Can you work these out from the model? Positions are in its coordinate system, mm. Face numbers are marked on the shaded views. A direction names the side the tool comes from. Round coordinates to 2 decimals unless told otherwise and drop trailing zeros. Order: outer loops, then holes, each group sorted by start corner. A loop starts at its lowest first (then second) coordinate and runs counter-clockwise, first axis right, second up. Notation, with made-up numbers: (2, -37) -> (60, -37) arc R16 ccw to (60, -26) -> close; hole circle Ø5 at (24, 66). An arc over 180 degrees is marked (long way). One line per item, written item: value.
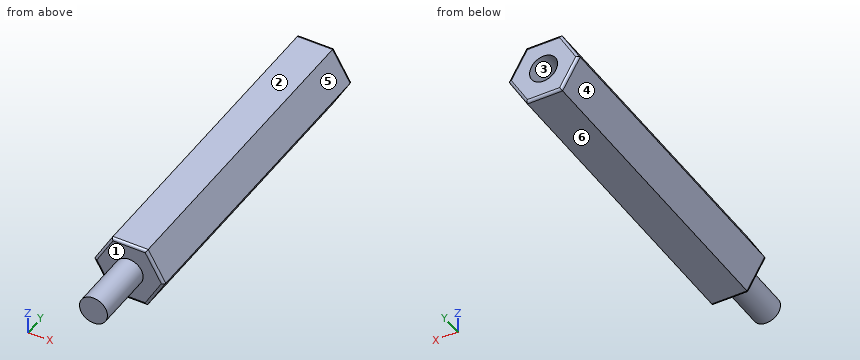
```python
from build123d import *

# Parameters (mm, degrees)
RESSALTO_EXTRUS_O1_DEPTH = 25
FILETE1_R                = 0.2
ESBO_O2_R                = 1.0922
RESSALTO_EXTRUS_O2_DEPTH = 4.76
ESBO_O3_R                = 1.0922
CORTE_EXTRUS_O1_DEPTH    = 4.76


with BuildPart() as part:
    # Esboço1 → Ressalto-extrusão1 (new body)
    with BuildSketch(Plane(origin=(0, 0, 0), x_dir=(1, 0, 0), z_dir=(0, 1, 0))):
        Polygon((2.748187281, 0), (1.374093641, 2.38), (-1.374093641, 2.38), (-2.748187281, 0), (-1.374093641, -2.38), (1.374093641, -2.38), align=None)
    extrude(amount=RESSALTO_EXTRUS_O1_DEPTH)

    # Filete1
    filete1_edges = [part.edges().sort_by_distance(p)[0] for p in [
        (0, 25, -2.38),
        (-2.061140461, 25, -1.19),
        (-2.061140461, 25, 1.19),
        (0, 25, 2.38),
        (2.061140461, 25, 1.19),
        (0, 0, 2.38),
        (-2.061140461, 0, 1.19),
        (-2.061140461, 0, -1.19),
        (2.061140461, 25, -1.19),
        (0, 0, -2.38),
        (2.061140461, 0, -1.19),
        (2.061140461, 0, 1.19),
    ]]
    fillet(filete1_edges, radius=FILETE1_R)

    # Esboço2 → Ressalto-extrusão2 (add)
    with BuildSketch(Plane.XZ):
        Circle(ESBO_O2_R)
    extrude(amount=RESSALTO_EXTRUS_O2_DEPTH)

    # Esboço3 → Corte-extrusão1 (cut)
    with BuildSketch(Plane(origin=(0, 25, 0), x_dir=(1, 0, 0), z_dir=(0, 1, 0))):
        Circle(ESBO_O3_R)
    extrude(amount=-CORTE_EXTRUS_O1_DEPTH, mode=Mode.SUBTRACT)


solid = part.part
```
Q1. Please list where these lines run through material, in increasing order: line 1 along Z through (x, y) = (0, 21.55); line 2 along Y through (x, z) = (-2.15, -0.5); line 3 along Z through (x, y) = (0.75, 23).
Answers below:
line 1: -2.38 to -1.09, 1.09 to 2.38
line 2: 0 to 25
line 3: -2.38 to -0.79, 0.79 to 2.38
Q2. I want a section at A-A on x = 0. List the corners of the cut face in (y, z) for me, plus the area to 3 significant figures.
Answers below:
outline: (-4.76, -1.09) -> (0, -1.09) -> (0, -2.18) arc R0.2 ccw to (0.2, -2.38) -> (24.8, -2.38) arc R0.2 ccw to (25, -2.18) -> (25, -1.09) -> (20.24, -1.09) -> (20.24, 1.09) -> (25, 1.09) -> (25, 2.18) arc R0.2 ccw to (24.8, 2.38) -> (0.2, 2.38) arc R0.2 ccw to (0, 2.18) -> (0, 1.09) -> (-4.76, 1.09) -> close
area: 119 mm^2
Q3. I want a section at B-B on y = 19.75. List the corners of the cut face in (x, z) for me, plus the area to 3 significant figures.
Answers below:
outline: (-2.75, 0) -> (-1.37, -2.38) -> (1.37, -2.38) -> (2.75, 0) -> (1.37, 2.38) -> (-1.37, 2.38) -> close
area: 19.6 mm^2
Q4. We'd pull the mould along X, two halves only. Please class the marked faces 3, 4, 5 and 6: released by +X, released by -X, zero draft, split by the parting line, or undercut.
Answers below:
face 3: undercut
face 4: released by -X
face 5: released by +X
face 6: zero draft
Q5. On a 3-axis mill with a long thin cutter (end or side, diameter ignored), from which of +Z, -Z, +X, -X, +Y, -Y can I reach the whole of each face in a straight line? I mean the marked faces 1 and 2. Say none if no direction works.
Answers below:
face 1: -Y
face 2: +Z, +X, -X, +Y, -Y
Q6. Will this pin go through, and if not, where does the flat tip stop? pin 1 Ø1.7 at (x, z) = (0.5, -0.5) entering from +Y.
Answers below:
pin 1: y = 25
